from build123d import *

# Parameters (mm, degrees)
F0_W      = 86.36
F0_H      = 58.42
F1_DEPTH  = 61.722
F2_W      = 13.0146164447
F2_H      = 11.5111361851
F2_W_2    = 9.3842569146
F2_H_2    = 7.7007600234
F3_DEPTH  = 56.642
F4_W      = 81.28
F4_H      = 55.88
F5_DEPTH  = 55.88
F6_W      = 81.28
F6_H      = 2.3422017694
F7_DEPTH  = 55.88
F8_W      = 10.16
F8_H      = 49.7436418003
F8_H_2    = 8.6763581997
F9_DEPTH  = 3.556
F10_W     = 7.5672202845
F10_H     = 1.6030113697
F10_H_2   = 0.9847168326
F11_DEPTH = 69.342
F12_DEPTH = 7.366
F13_W     = 7.66663257
F13_H     = 26.7714005868
F14_DEPTH = 55.88
F15_W     = 7.66663257
F15_H     = 26.7663976438
F16_DEPTH = 55.88
F17_W     = 17.341342
F17_H     = 15.24
F18_DEPTH = 25.4


with BuildPart() as f1:
    # F0 (on Front) → F1 (new body)
    with BuildSketch(Plane.XZ):
        with Locations((-2.54, 0)):
            Rectangle(F0_W, F0_H)
    extrude(amount=-F1_DEPTH)

    # F2 (on face) → F3 (cut)
    with BuildSketch(Plane.XZ):
        Polygon((27.8808352199, 13.7387597933), (7.5608352199, 13.7387597933), (7.5608352199, 4.9298959784), (7.5608352199, -6.5812402067), (27.8808352199, -6.5812402067), (27.8808352199, 1.1195198167), align=None)
        with Locations((1.0535269976, -0.8256721141)):
            Rectangle(F2_W, F2_H)
        with Locations((32.5729636772, -2.730860195)):
            Rectangle(F2_W_2, F2_H_2)
    extrude(amount=-F3_DEPTH, mode=Mode.SUBTRACT)

    # F4 (on face) → F5 (cut)
    with BuildSketch(Plane.XY.offset(29.21)):
        with Locations((-2.54, 31.242)):
            Rectangle(F4_W, F4_H)
    extrude(amount=-F5_DEPTH, mode=Mode.SUBTRACT)

    # F6 (on face) → F7 (join)
    with BuildSketch(Plane.XY.offset(-26.67)):
        with Locations((-2.54, 31.2445014715)):
            Rectangle(F6_W, F6_H)
    extrude(amount=F7_DEPTH)

    # F8 (on face) → F9 (join)
    with BuildSketch(Plane(origin=(0, 61.722, 0), x_dir=(-1, 0, 0), z_dir=(0, 1, 0))):
        with Locations((2.54, -4.3381790999)):
            Rectangle(F8_W, F8_H)
        with Locations((2.54, 24.8718209001)):
            Rectangle(F8_W, F8_H_2)
    extrude(amount=F9_DEPTH)

    # F10 (on face) → F11 (cut)
    with BuildSketch(Plane.XY.offset(29.21)):
        with Locations((-2.54, 63.5)):
            Rectangle(F10_W, F10_H)
        with Locations((-2.54, 62.2061358988)):
            Rectangle(F10_W, F10_H_2)
    extrude(amount=-F11_DEPTH, mode=Mode.SUBTRACT)

    # F12 (add): a face of the model
    f12_faces = [f1.faces().sort_by_distance(p)[0] for p in [
        (-45.72, 30.861, 0),
    ]]
    extrude(f12_faces, amount=F12_DEPTH)

    # F13 (on face) → F14 (cut)
    with BuildSketch(Plane.XY.offset(29.21)):
        with Locations((-47.013316285, 16.6877002934)):
            Rectangle(F13_W, F13_H)
    extrude(amount=-F14_DEPTH, mode=Mode.SUBTRACT)

    # F15 (on face) → F16 (cut)
    with BuildSketch(Plane.XY.offset(29.21)):
        with Locations((-47.013316285, 45.7988011781)):
            Rectangle(F15_W, F15_H)
    extrude(amount=-F16_DEPTH, mode=Mode.SUBTRACT)

    # F17 (on face) → F18 (cut)
    with BuildSketch(Plane(origin=(-53.086, 0, 0), x_dir=(0, -1, 0), z_dir=(-1, 0, 0))):
        with Locations((-14.1710711635, 1.3578335623)):
            Rectangle(F17_W, F17_H)
    extrude(amount=-F18_DEPTH, mode=Mode.SUBTRACT)


solid = f1.part
Read the model definition and answer for the solid it produces. Units are mm, in the model's axes. A direction names the side the tool comes from. Round coordinates to 2 decimals unless told otherwise and drop trailing zeros. Write each loop counter-clockwise with the first axis right and the second up, starting at its lowest first coordinate (ties: lowest second). Pieces come first, ordered by that corner, then holes.
Q1. Find section A-A on z = -2.5. Determine the outline of the cut face in (x, y).
Values:
outline: (-53.09, 0) - (-5.45, 0) - (-5.45, 3.3) - (-50.85, 3.3) - (-50.85, 5.5) - (-53.09, 5.5) - close; (-53.09, 22.84) - (-50.85, 22.84) - (-50.85, 30.07) - (38.1, 30.07) - (38.1, 3.3) - (37.27, 3.3) - (37.27, 0) - (40.64, 0) - (40.64, 61.72) - (2.54, 61.72) - (2.54, 65.28) - (-7.62, 65.28) - (-7.62, 61.72) - (-53.09, 61.72) - close; hole (-50.85, 32.42) - (38.1, 32.42) - (38.1, 59.18) - (-50.85, 59.18) - close; hole (-6.32, 61.71) - (1.24, 61.71) - (1.24, 64.3) - (-6.32, 64.3) - close
Q2. Flat-ended cylindrical pins translate along their axes: P1, Ø3, axis at x = -37.5, z = 12, coming from the +Y side; P2, Ø2.5, axis at x = -2, z = -5, coming from the -Y side; P3, Ø4, axis at y = 64, z = 0.5, coming from the -X side. Find the tip coordinate at first contact, or state that the pin passes through.
Values:
P1: stops at y = 61.72
P2: stops at y = 30.07
P3: stops at x = -7.62
Q3. Straight lines are drawn through the part: line 1 (Y direction, x = -2.5, z = -0.5); line 2 (Y direction, x = 8, z = -14); line 3 (Y direction, x = -3, z = 11.5). For each, find the intervals that lie inside material, in ascending order.
Values:
line 1: y = 30.07 to 32.42, 59.18 to 61.71, 64.3 to 65.28
line 2: y = 0 to 3.3, 30.07 to 32.42, 59.18 to 61.72
line 3: y = 0 to 3.3, 30.07 to 32.42, 59.18 to 61.71, 64.3 to 65.28
Q4. Find section C-C on y = 20.5. Determine the outline of the cut face in (x, z).
Values:
outline: (-53.09, -29.21) - (40.64, -29.21) - (40.64, 29.21) - (38.1, 29.21) - (38.1, -26.67) - (-50.85, -26.67) - (-50.85, -6.26) - (-53.09, -6.26) - close; (-53.09, 8.98) - (-50.85, 8.98) - (-50.85, 29.21) - (-53.09, 29.21) - close
Q5. Find section D-D on z = 25.5. Determine the outline of the cut face in (x, y), and give its area (3 significant figures).
Values:
outline: (-53.09, 0) - (40.64, 0) - (40.64, 61.72) - (2.54, 61.72) - (2.54, 65.28) - (-7.62, 65.28) - (-7.62, 61.72) - (-53.09, 61.72) - close; hole (-50.85, 3.3) - (38.1, 3.3) - (38.1, 30.07) - (-50.85, 30.07) - close; hole (-50.85, 32.42) - (38.1, 32.42) - (38.1, 59.18) - (-50.85, 59.18) - close; hole (-6.32, 61.71) - (1.24, 61.71) - (1.24, 64.3) - (-6.32, 64.3) - close
area: 1,040 mm2
Q6. Find section B-B on x = 32.5. Determine the outline of the cut face in (y, z), and give its area (3 significant figures).
Values:
outline: (0, -29.21) - (61.72, -29.21) - (61.72, 29.21) - (59.18, 29.21) - (59.18, -26.67) - (32.42, -26.67) - (32.42, 29.21) - (30.07, 29.21) - (30.07, -26.67) - (3.3, -26.67) - (3.3, -6.58) - (0, -6.58) - close; (0, 1.12) - (3.3, 1.12) - (3.3, 29.21) - (0, 29.21) - close
area: 589 mm2
Q7. A tool of negligible diameter and unlimited length cuts with its end or side. For faces 4 (the face through (-7.62, 63, 0)), 5 (the face through (-5.454, 2, -1)), 6 (the face through (-7, 32.416, 2)), from which of +Z, -Z, +X, -X, +Y, -Y can it reach the whole face along a straight path? Write none if from no direction.
Values:
face 4: +Z, -Z, -X, +Y
face 5: -Y
face 6: +Z
Q8. The mould has two halves that part along Y. Classify faces 1 (the face through (-30, 61.722, 0)), 2 (the face through (-53.086, 30, 0)), 3 (the face through (-50.847, 25, 2)): released by +Y, released by -Y, zero draft, split by the parting line, or undercut.
Values:
face 1: released by +Y
face 2: zero draft
face 3: undercut
